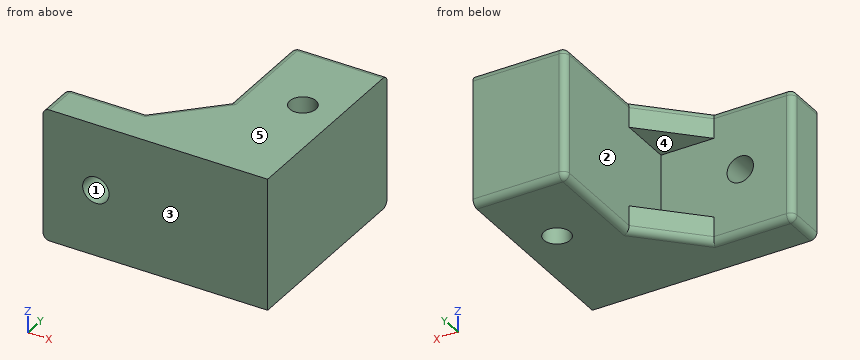
from build123d import *

# Parameters (mm, degrees)
ESQUISSE2_W                  = 7
ESQUISSE2_H                  = 10
BOSS_EXTRU_1_DEPTH           = 15
ESQUISSE3_W                  = 10
ESQUISSE3_H                  = 3
BOSS_EXTRU_2_DEPTH           = 10
BOSS_EXTRU_3_DEPTH           = 2
ESQUISSE7_R                  = 1
ENL_V_MAT_EXTRU_1_DEPTH      = 13
ENL_V_MAT_EXTRU_1_DEPTH_BACK = 4
ESQUISSE8_R                  = 1
ENL_V_MAT_EXTRU_2_DEPTH      = 1
ENL_V_MAT_EXTRU_2_DEPTH_BACK = 11
CONG_1_R                     = 0.5


with BuildPart() as part:
    # Esquisse2 → Boss.-Extru.1 (new body)
    with BuildSketch(Plane(origin=(0, 0, 0), x_dir=(1, 0, 0), z_dir=(0, 1, 0))):
        Rectangle(ESQUISSE2_W, ESQUISSE2_H)
    extrude(amount=BOSS_EXTRU_1_DEPTH)

    # Esquisse3 → Boss.-Extru.2 (add)
    with BuildSketch(Plane.ZY.offset(3.5)):
        with Locations((0, 1.5)):
            Rectangle(ESQUISSE3_W, ESQUISSE3_H)
    extrude(amount=BOSS_EXTRU_2_DEPTH)

    # Esquisse6 → Boss.-Extru.3 (add)
    with BuildSketch(Plane.XY.offset(5)):
        Polygon((-7.5, 3), (-3.5, 7), (-3.5, 3), align=None)
    boss_extru_3 = extrude(amount=-BOSS_EXTRU_3_DEPTH)

    # Symétrie1: Boss.-Extru.3 across plane
    add(boss_extru_3.mirror(Plane.XY))

    # Esquisse7 → Enlèv. mat.-Extru.1 (cut, two sides)
    with BuildSketch(Plane(origin=(0, 3, 0), x_dir=(1, 0, 0), z_dir=(0, 1, 0))) as enl_v_mat_extru_1_sk:
        with Locations((-9.5, 0)):
            Circle(ESQUISSE7_R)
    extrude(amount=ENL_V_MAT_EXTRU_1_DEPTH, mode=Mode.SUBTRACT)
    extrude(enl_v_mat_extru_1_sk.sketch, amount=-ENL_V_MAT_EXTRU_1_DEPTH_BACK, mode=Mode.SUBTRACT)

    # Esquisse8 → Enlèv. mat.-Extru.2 (cut, two sides)
    with BuildSketch(Plane.XY.offset(5)) as enl_v_mat_extru_2_sk:
        with Locations((0.75, 9)):
            Circle(ESQUISSE8_R)
    extrude(amount=ENL_V_MAT_EXTRU_2_DEPTH, mode=Mode.SUBTRACT)
    extrude(enl_v_mat_extru_2_sk.sketch, amount=-ENL_V_MAT_EXTRU_2_DEPTH_BACK, mode=Mode.SUBTRACT)

    # Congé1
    cong_1_edges = [part.edges().sort_by_distance(p)[0] for p in [
        (0, 15, -5),
        (-10.5, 3, -5),
        (-10.5, 3, 5),
        (-13.5, 1.5, -5),
        (-13.5, 1.5, 5),
        (-13.5, 3, 0),
        (-5.5, 5, 5),
        (-3.5, 15, 0),
        (-5.5, 5, -5),
        (0, 15, 5),
        (-3.5, 11, -5),
        (-3.5, 11, 5),
    ]]
    fillet(cong_1_edges, radius=CONG_1_R)


solid = part.part
Geometry check sheet. Reference: the model listing, model coordinates, mm. Face numbers are marked on the shaded views. A direction names the side the tool comes from. Give positions to 0.01 mm unless a question says otherwise; leave off trailing zeros. Loops run counter-clockwise (first coordinate to the right, second up) from the corner with the lowest first, then second, coordinate; pieces in that order, holes last. Notation, with made-up numbers: M 31.5,-3 L 42.5,-3 A7 cw 42.5,4 Z; hole C 72.25,47.5 d1. An arc over 180 degrees is marked long. Answer as a JSON object with one key per item and string values. Group by question number.
Item 1: Sectioned sample at D-D on z = -1.5. Record the boundary of the cut face in (x, y).
Item 2: Access from +Z, -Z, +X, -X, +Y, -Y to the whole of each face (thin tool, end or side, straight path). Record for the marked faces 4 and 5.
Item 3: Sectioned sample at B-B on y = 9. Record the boundary of the cut face in (x, z).
Item 4: Gauge pin test, flat ends, axial feed: pin 1 (2 mm diameter, centred on x = -6, y = 6, fed in from -Z); pin 2 (4.5 mm diameter, centred on y = 10.5, z = -0.5, fed in from -X). Record the tip position at first contact, or that the pin passes through.
Item 5: Sectioned sample at C-C on x = 0.75. Record the boundary of the cut face in (y, z).
Item 6: Mould release check, pull along X, two halves, no side actions. Record for the marked faces 1, 2 and 3: pulls with the +X half, pulls with the -X half, needs draft (parallel to the pull), parting line crosses it, or undercut.
Item 7: Sectioned sample at A-A on z = 0. Record the boundary of the cut face in (x, y).
Item 8: Material ranges on L1, parallel to Z at x = -9.5, y = 1.85; L2, parallel to X at y = 1.8, z = 0; L3, parallel to Y at x = 0.75, z = 1, recorded low to high.
Findings below:
{
 "1": {"outline": "M -13.5,0 L 3.5,0 L 3.5,15 L -3,15 A0.5 ccw -3.5,14.5 L -3.5,3 L -13,3 A0.5 ccw -13.5,2.5 Z; hole C 0.75,9 d2"},
 "2": {"face 4": "-X, +Y", "face 5": "+Z, +X, -X, +Y, -Y"},
 "3": {"outline": "M -3.5,-4.5 A0.5 ccw -3,-5 L -0.25,-5 L -0.25,5 L -3,5 A0.5 ccw -3.5,4.5 Z; M 1.75,-5 L 3.5,-5 L 3.5,5 L 1.75,5 Z"},
 "4": {"pin 1": "through", "pin 2": "x = -3.5"},
 "5": {"outline": "M 0,-5 L 8,-5 L 8,5 L 0,5 Z; M 10,-5 L 14.5,-5 A0.5 ccw 15,-4.5 L 15,4.5 A0.5 ccw 14.5,5 L 10,5 Z"},
 "6": {"face 1": "undercut", "face 2": "pulls with the -X half", "face 3": "needs draft"},
 "7": {"outline": "M -13.5,0 L -10.5,0 L -10.5,3 L -13,3 A0.5 ccw -13.5,2.5 Z; M -8.5,0 L 3.5,0 L 3.5,15 L -3,15 A0.5 ccw -3.5,14.5 L -3.5,3 L -8.5,3 Z; hole C 0.75,9 d2"},
 "8": {"L1": "-5 to -1, 1 to 5", "L2": "-13.5 to -10.5, -8.5 to 3.5", "L3": "0 to 8, 10 to 15"}
}
